Model file for the job. Use its own axes, mm. A direction names the side the tool comes from. Round coordinates to 2 decimals unless told otherwise and drop trailing zeros. Write each loop counter-clockwise with the first axis right and the second up, starting at its lowest first coordinate (ties: lowest second). Pieces come first, ordered by that corner, then holes. Notation, with made-up numbers: (47.25, 79) - (61.25, 79) arc R24 cw to (61.25, 96) - close; hole circle Ø6 at (-9.5, -26.75). An arc over 180 degrees is marked (long way). Answer as a JSON object with one key per item and string values. Group by question number.
from build123d import *

# Parameters (mm, degrees)
F0_W        = 25
F0_H        = 120
F1_DEPTH    = 13.5
F2_R        = 3.1
F3_DEPTH    = 13.501
F4_W        = 13
F4_H        = 17.8598619506
F5_DEPTH    = 12.5
F6_R        = 3.325
F7_DEPTH    = 4.2
F8_T        = 3.5
F8_T3_DEPTH = 19.5
F8_T5_DEPTH = 23
F8_T7_DEPTH = 20
F8_T9_DEPTH = 23


# Not quite as in the source:
# - a shell that OpenCascade refuses in one call is made with other operations: the cavity is built on its own and cut out


with BuildPart() as f1:
    # F0 (on Front) → F1 (new body)
    with BuildSketch(Plane.XZ):
        Rectangle(F0_W, F0_H)
    extrude(amount=F1_DEPTH)

    # F2 (on face) → F3 (cut, through all)
    with BuildSketch(Plane.XZ.offset(13.5)):
        Circle(F2_R)
    extrude(amount=-F3_DEPTH, mode=Mode.SUBTRACT)

    # F4 (on face) → F5 (cut)
    with BuildSketch(Plane(origin=(0, 0, 0), x_dir=(-1, 0, 0), z_dir=(0, 1, 0))):
        with Locations((0, 52.9299309753)):
            Rectangle(F4_W, F4_H)
        with Locations((0, -52.9299309753)):
            Rectangle(F4_W, F4_H)
    extrude(amount=-F5_DEPTH, mode=Mode.SUBTRACT)

    # F6 (on face) → F7 (cut)
    with BuildSketch(Plane.XZ.offset(13.5)):
        with Locations((0, -40.5)):
            Circle(F6_R)
        with Locations((0, 40.5)):
            Circle(F6_R)
    extrude(amount=-F7_DEPTH, mode=Mode.SUBTRACT)

    # F8: shell of thickness 3.5, made by hand


with BuildPart() as f8_core1:
    # F8_t2: copy of F1
    add(f1.part)

    # the walls: a layer under each face that stays
    f8_faces = [f8_core1.faces().sort_by_distance(p)[0] for p in [
        (12.5, -6.75, 0),
        (-8.3333333333, -11.25, -60),
        (8.3333333333, -11.25, 60),
        (-8.3333333333, -13.5, -40),
        (-6.5, -6.25, -52),
        (0, -12.5, -52),
        (6.5, -6.25, -52),
        (-12.5, -6.75, 0),
        (6.5, -6.25, 52),
        (0, -12.5, 52),
        (-6.5, -6.25, 52),
        (0, -6.25, -44),
        (0, -6.25, 44),
        (-3.1, -6.75, 0),
        (-3.325, -11.4, -40.5),
        (-3.325, -11.4, 40.5),
        (0, -9.3, -40.5),
        (0, -9.3, 40.5),
    ]]
    thicken(f8_faces, amount=-F8_T, mode=Mode.SUBTRACT)

    # F8_s4 → F8_t3 (cut)
    with BuildSketch(Plane.XZ.offset(-3.5)):
        Polygon((-6.465, -44.035), (-10, -44), (-10, -40.5), (-6.5, -40.5), align=None)
        Polygon((6.465, -44.035), (10, -44), (10, -40.5), (6.5, -40.5), align=None)
        Polygon((6.465, 44.035), (10, 44), (10, 40.5), (6.5, 40.5), align=None)
        Polygon((-6.465, 44.035), (-10, 44), (-10, 40.5), (-6.5, 40.5), align=None)
    extrude(amount=F8_T3_DEPTH, mode=Mode.SUBTRACT)

    # F8_s6 → F8_t5 (cut)
    with BuildSketch(Plane.XY.offset(-63.5)):
        Polygon((-6.465, -12.465), (-10, -12.5), (-10, -16), (-6.5, -16), align=None)
        Polygon((6.465, -12.465), (6.5, -16), (10, -16), (10, -12.5), align=None)
    extrude(amount=F8_T5_DEPTH, mode=Mode.SUBTRACT)

    # F8_s8 → F8_t7 (cut)
    with BuildSketch(Plane.YZ.offset(-10)):
        Polygon((-12.465, -44.035), (-16, -44), (-16, -40.5), (-12.5, -40.5), align=None)
        Polygon((-12.465, 44.035), (-16, 44), (-16, 40.5), (-12.5, 40.5), align=None)
    extrude(amount=F8_T7_DEPTH, mode=Mode.SUBTRACT)

    # F8_s10 → F8_t9 (cut)
    with BuildSketch(Plane.XY.offset(40.5)):
        Polygon((6.465, -12.465), (10, -12.5), (10, -16), (6.5, -16), align=None)
        Polygon((-6.465, -12.465), (-6.5, -16), (-10, -16), (-10, -12.5), align=None)
    extrude(amount=F8_T9_DEPTH, mode=Mode.SUBTRACT)

    # F8_s11 → F8_t12 (revolve, cut)
    with BuildSketch(Plane.XY.offset(-40.5)):
        Polygon((3.29, -9.335), (6.825, -9.3), (6.825, -5.8), (3.325, -5.8), align=None)
    revolve(axis=Axis((0, -9.3, -40.5), (0, -1, 0)), mode=Mode.SUBTRACT)

    # F8_s13 → F8_t14 (revolve, cut)
    with BuildSketch(Plane.XY.offset(40.5)):
        Polygon((3.29, -9.335), (6.825, -9.3), (6.825, -5.8), (3.325, -5.8), align=None)
    revolve(axis=Axis((0, -9.3, 40.5), (0, -1, 0)), mode=Mode.SUBTRACT)


with BuildPart() as f1_1:
    add(f1.part)

    # what is left inside the walls is the cavity
    f8_cavity = [f8_core1.part.solids().sort_by_distance(p)[0] for p in [
        (0, -0.035, -13.5),
    ]]
    add(f8_cavity, mode=Mode.SUBTRACT)


solid = f1_1.part
(1) Flat gauge pins, fed straight in: pin 1 (6.5 mm diameter, centred on x = 2.5, z = -48.5, fed in from +Y); pin 2 (3 mm diameter, centred on x = 2.5, y = -4.5, fed in from +Z); pin 3 (7.5 mm diameter, centred on x = -3.5, z = -36.5, fed in from +Y); pin 4 (8 mm diameter, centred on x = 0, z = 0, fed in from -Y). Where does each tip first touch, or does it go through?
(2) Slice it at A-A (y = -4.25). Write the cut outline in (x, z), then the cut area to 3 significant figures.
(3) Slice it at D-D (z = -16). Write the cut outline in (x, y), then the cut area to 4 significant figures.
(4) Pull direction Z, two halves, no side cores. Call faces 1 (the flat face through (0, -6, 44)), 2 (the flat face through (0, -9.3, -40)), 3 (the cylindrical face through (-0.4, -11.4, -37.2)), 4 (the flat face through (-12.5, -7, -1)): pulls with the +Z half, pulls with the -Z half, needs draft (parallel to the pull), parting line crosses it, or undercut.
(5) Slice it at B-B (z = 0). Write the cut outline in (x, y).
(6) 3-axis set-ups, long thin cutter, end or side, ignore diameter. For faces 5 (the flat face through (9, -5, -1)), 6 (the flat face through (0, -12.5, 52)), 7 (the flat face through (0, -12.5, -52)), 8 (the flat face through (0, -13, -60)), 9 (the flat face through (0, -13, 60)): which of +Z, -Z, +X, -X, +Y, -Y reach the whole face in a straight line?
(7) Drill centre lines: line 1 (Z direction, x = 0, y = -11.65) (3 decimals); line 2 (Z direction, x = 0, y = -6) (3 decimals); line 3 (X direction, y = -11.5, z = -47.5). Where is each one in solid material? Low to high. Write a range as from..to.
Answer:
{
 "1": {"pin 1": "y = -12.5", "pin 2": "z = 44", "pin 3": "y = -5.8", "pin 4": "y = -13.5"},
 "2": {"outline": "(-12.5, -60) - (-6.5, -60) - (-6.5, -44) - (6.5, -44) - (6.5, -60) - (12.5, -60) - (12.5, 60) - (6.5, 60) - (6.5, 44) - (-6.5, 44) - (-6.5, 60) - (-12.5, 60) - close; circle Ø13.2 at (0, 0); hole (-9, -40.5) - (9, -40.5) - (9, 40.5) - (-9, 40.5) - close; hole circle Ø6.2 at (0, 0)", "area": "1,230 mm²"},
 "3": {"outline": "(-12.5, -13.5) - (12.5, -13.5) - (12.5, 0) - (9, 0) - (9, -10) - (-9, -10) - (-9, 0) - (-12.5, 0) - close", "area": "157.5 mm²"},
 "4": {"face 1": "pulls with the +Z half", "face 2": "undercut", "face 3": "undercut", "face 4": "needs draft"},
 "5": {"outline": "(-12.5, -13.5) - (-3.1, -13.5) - (-3.1, 0) - (-6.6, 0) - (-6.6, -10) - (-9, -10) - (-9, 0) - (-12.5, 0) - close; (3.1, -13.5) - (12.5, -13.5) - (12.5, 0) - (9, 0) - (9, -10) - (6.6, -10) - (6.6, 0) - (3.1, 0) - close"},
 "6": {"face 5": "+Y", "face 6": "+Z, +Y", "face 7": "-Z, +Y", "face 8": "-Z, +X, -X, +Y, -Y", "face 9": "+Z, +X, -X, +Y, -Y"},
 "7": {"line 1": "-44..-43.825, -37.175..-3.1, 3.1..37.175, 43.825..44", "line 2": "-44..-33.675, -6.6..-3.1, 3.1..6.6, 33.675..44", "line 3": "-12.5..-6.5, 6.5..12.5"}
}
